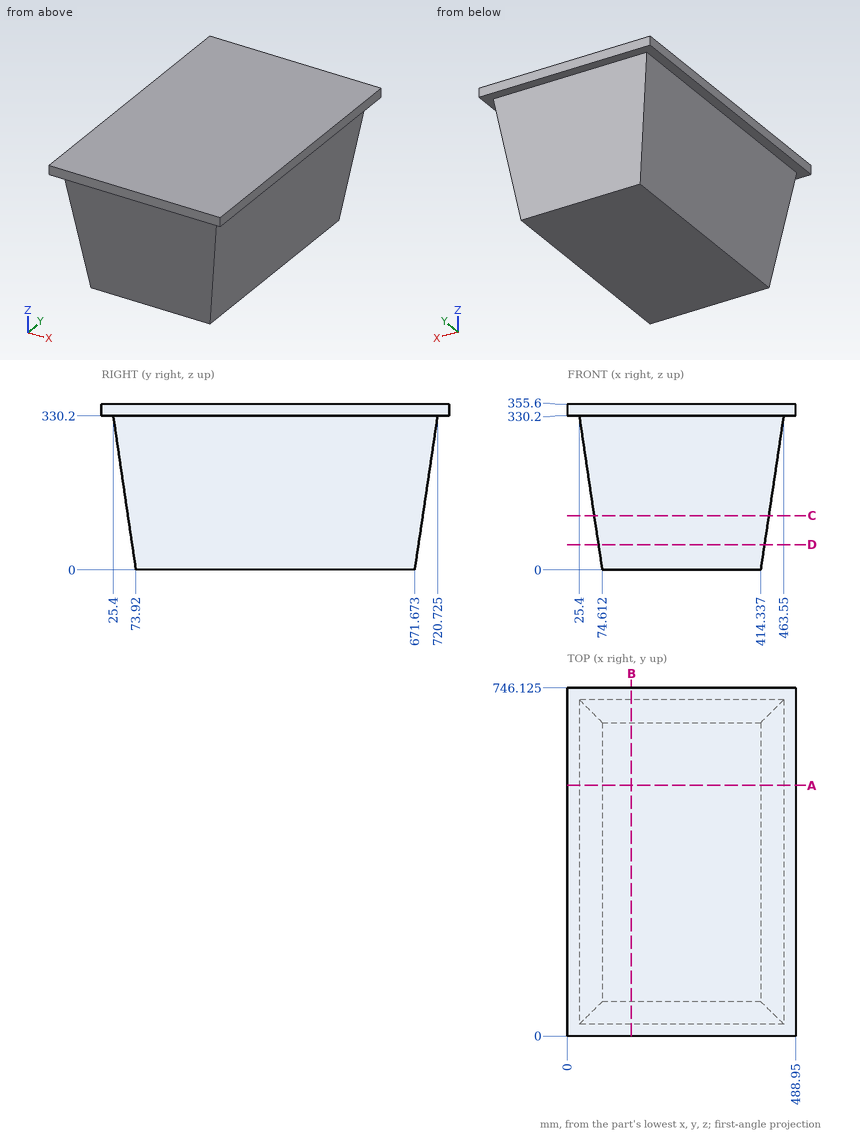
Answer from the drawing. Dimensions are ordinates in mm from the lowest x, y and z of the part. Round coordinates to 2 decimals unless told otherwise and drop trailing zeros. Loops run counter-clockwise (first coordinate to the right, second up) from the corner with the lowest first, then second, coordinate; pieces in that order, holes last. Notation, with made-up numbers: (16, 59) - (31, 59) arc R15 ccw to (31, 88) - close; hole circle Ø3 at (3.5, 72). An arc over 180 degrees is marked (long way). One line per item, written item: value.
Q1. Find section A-A on y = 537. Give the vertices of the cut face in (x, z), and give its area (3 significant figures).
Check values:
outline: (0, 330.2) - (25.4, 330.2) - (74.61, 0) - (414.34, 0) - (463.55, 330.2) - (488.95, 330.2) - (488.95, 355.6) - (0, 355.6) - close
area: 141,000 mm2
Q2. Find section C-C on z = 116.5. Give the vertices of the cut face in (x, y).
Check values:
outline: (57.25, 56.8) - (431.7, 56.8) - (431.7, 688.98) - (57.25, 688.98) - close
Q3. Straight lines are drawn through the part: probe 1 along X at (y, z) = (487, 330); probe 2 along X at (y, z) = (324, 51); probe 3 along Y at (x, z) = (254, 145). For each, find the intervals that lie inside material, in ascending order.
Check values:
probe 1: 25.43 to 463.52
probe 2: 67.01 to 421.94
probe 3: 52.61 to 693.21
Q4. Find section B-B on x = 137. Give the vertices of the cut face in (y, z) (1 decimal), and give its area (3 significant figures).
Check values:
outline: (0, 330.2) - (25.4, 330.2) - (73.9, 0) - (671.7, 0) - (720.7, 330.2) - (746.1, 330.2) - (746.1, 355.6) - (0, 355.6) - close
area: 232,000 mm2
Q5. Each of these flat-tipped pins is pushed along its axis until it touches: pin 1 Ø1 at (x, z) = (407.5, 150.5) entering from -Y; pin 2 Ø12 at (x, z) = (56.5, 156) entering from -Y (1 decimal); pin 3 Ø5 at (y, z) = (133.5, 58.5) entering from +X. Where does it stop, or does it pass through?
Check values:
pin 1: y = 51.73
pin 2: y = 50.1
pin 3: x = 423.43
Q6. Find section D-D on z = 54. Give the vertices of the cut face in (x, y) (1 decimal), and give its area (3 significant figures).
Check values:
outline: (66.6, 66) - (422.4, 66) - (422.4, 679.7) - (66.6, 679.7) - close
area: 218,000 mm2
